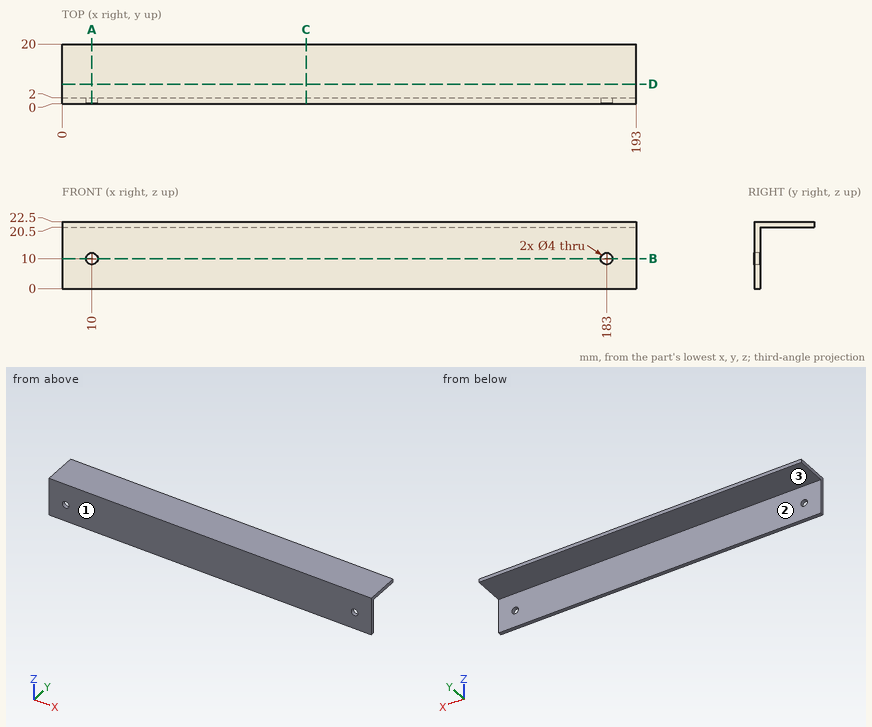
For this review, use the dimensioned drawing (mm, ordinates from the lowest corner) and the shaded views. Give positions to 0.01 mm unless a question says otherwise; leave off trailing zeros. Order: outer loops, then holes, each group sorted by start corner. A loop starts at its lowest first (then second) coordinate and runs counter-clockwise, first axis right, second up. Notation, with made-up numbers: (62.5, -34) - (87.5, -34) arc R28 ccw to (87.5, -4) - close; hole circle Ø11 at (62, 23.5). An arc over 180 degrees is marked (long way). Write item = value, one per line. Start each with the question number.
Q1. Mouldability with a two-part tool opening along Y and no side actions: class the marked faces 1, 2 and 3 as released by +Y, released by -Y, zero draft, split by the parting line, or undercut.
Q2. To check wall thickness, follow L1, parallel to X at y = 1.25, z = 10; L2, parallel to Z at x = 183, y = 1.45; L3, parallel to Y at x = 51, z = 12.5. State the ranges of each line that lie inside material, in increasing order. Write a range as from..to.
Q3. Clearance check with flat-ended pins moving along their axes: pin 1 Ø1.5 at (x, y) = (27.5, 3.5) entering from -Z; pin 2 Ø2.5 at (x, z) = (183, 10) entering from -Y; pin 3 Ø4 at (x, z) = (49.5, 3) entering from +Y. State where each tip first meets the part, or that it passes through.
Q4. We need section D-D on y = 6.5. State the section outline as (x, z) points.
Q5. We need section C-C on x = 82. State the section outline as (y, z) points, plus the area to 3 significant figures.
Q6. We need section A-A on x = 10. State the section outline as (y, z) points.
Q7. We need section B-B on z = 10. State the section outline as (x, y) points, plus the area to 3 significant figures.
Working result:
q1.face_1 = released by -Y
q1.face_2 = released by +Y
q1.face_3 = zero draft
q2.L1 = 0..8, 12..181, 185..193
q2.L2 = 0..8, 12..22.5
q2.L3 = 0..2
q3.pin_1 = 20.5
q3.pin_2 = through
q3.pin_3 = 2
q4.outline = (0, 20.5) - (193, 20.5) - (193, 22.5) - (0, 22.5) - close
q5.outline = (0, 0) - (2, 0) - (2, 20.5) - (20, 20.5) - (20, 22.5) - (0, 22.5) - close
q5.area = 81.0 mm²
q6.outline = (0, 0) - (2, 0) - (2, 8) - (0, 8) - close; (0, 12) - (2, 12) - (2, 20.5) - (20, 20.5) - (20, 22.5) - (0, 22.5) - close
q7.outline = (0, 0) - (8, 0) - (8, 2) - (0, 2) - close; (12, 0) - (181, 0) - (181, 2) - (12, 2) - close; (185, 0) - (193, 0) - (193, 2) - (185, 2) - close
q7.area = 370 mm²
